The listing builds one solid part. Answer for the finished solid, in the listing's coordinates (mm). A direction names the side the tool comes from. Give positions to 0.01 mm unless a question says otherwise; leave off trailing zeros. Loops run counter-clockwise (first coordinate to the right, second up) from the corner with the lowest first, then second, coordinate; pieces in that order, holes last. Notation, with made-up numbers: (-26.75, 9.5) - (22.25, 9.5) arc R23 ccw to (22.25, 39.5) - close; hole circle Ø10 at (57, -14). An arc over 180 degrees is marked (long way). Write item = value, one per line. Start each with the question number.
1) Consider probe 1 along X at (y, z) = (69, -5.5); probe 2 along X at (y, z) = (896.5, 0); probe 3 along Y at (x, z) = (-12.5, 2). Determine where each line is inside the solid, lowest interval first.
2) The part is cut by section A-A on y = 520. Write down the section's boundary in (x, z).
3) Which of the six approach directions +Z, -Z, +X, -X, +Y, -Y give full straight-line access (tool end or side, diameter ignored) to faces 1 (the flat face through (-5, 0, -5)), 2 (the cylindrical face through (-2.38, 690.2, -10.74))?
4) Flat-ended cylindrical pins translate along their axes: P1, Ø0.5, axis at x = 13, y = 350, coming from the -Z side; P2, Ø9.5, axis at x = 0, z = 0, coming from the +Y side; P3, Ø2.5, axis at x = -15.5, z = 1, coming from the +Y side; P4, Ø0.8, axis at x = 16.5, y = 1050, coming from the +Z side. Find the tip coordinate at first contact, or state that the pin passes through.
Solid Edge part; units mm, degrees
sketch "Sketch1" plane through (0, 0, 0) normal (0, -1, 0) x (1, 0, 0)
  circle A0 centre (0, 0) radius 11
extrude "Protrusion1" add sketch "Sketch1" against normal blind 1400
sketch "Sketch2" plane through (0, 700, 0) normal (-1, 0, 0) x (0, -1, 0)
  line L0 (-353, 5) -> (-353, -5)
  line L1 (-353, -5) -> (-347, -5)
  line L2 (-347, -5) -> (-347, 5)
  line L3 (-347, 5) -> (-353, 5)
extrude "ExtrudedCutout_6" cut sketch "Sketch2" along normal mid plane 270
sketch "Sketch3" plane through (0, 700, 0) normal (-1, 0, 0) x (0, -1, 0)
  line L0 (-347, -5) -> (-347, 5)
  line L1 (-347, 5) -> (-353, 5)
  line L2 (-353, 5) -> (-353, -5)
  line L3 (-353, -5) -> (-347, -5)
extrude "ExtrudedProtrusion_8" add sketch "Sketch3" along normal mid plane 40
sketch "Sketch4" plane through (0, 700, 0) normal (-1, 0, 0) x (0, -1, 0)
  line L0 (347, -5) -> (353, -5)
  line L1 (353, -5) -> (353, 5)
  line L2 (353, 5) -> (347, 5)
  line L3 (347, 5) -> (347, -5)
extrude "ExtrudedCutout_7" cut sketch "Sketch4" along normal mid plane 50
sketch "Sketch5" plane through (0, 700, 0) normal (-1, 0, 0) x (0, -1, 0)
  line L0 (353, -5) -> (353, 5)
  line L1 (353, 5) -> (347, 5)
  line L2 (347, 5) -> (347, -5)
  line L3 (347, -5) -> (353, -5)
extrude "ExtrudedProtrusion_9" add sketch "Sketch5" along normal mid plane 40
hole "Hole_1" at (0, 0, 0) direction (0, 1, 0) diameter 12 end up to next
fillet "Round_1" radius 2.5 8 edges at (14.899, 1053, 5) (14.899, 1047, 5) (14.899, 1053, -5) (14.899, 1047, -5) (-14.899, 1047, 5) (-14.899, 1053, 5) (-14.899, 1053, -5) (-14.899, 1047, -5)
fillet "Round_2" radius 2.5 8 edges at (-14.899, 353, 5) (-14.899, 347, 5) (-14.899, 353, -5) (-14.899, 347, -5) (14.899, 353, 5) (14.899, 347, 5) (14.899, 353, -5) (14.899, 347, -5)
Answer below:
q1.probe_1 = -9.53 to -2.4, 2.4 to 9.53
q1.probe_2 = -11 to -6, 6 to 11
q1.probe_3 = 347 to 353, 1047 to 1053
q2.outline = circle Ø22 at (0, 0); hole circle Ø12 at (0, 0)
q3.face_1 = +Z, -Z, +X, -X, -Y
q3.face_2 = none
q4.P1 = -5
q4.P2 = through
q4.P3 = 1053
q4.P4 = 5
